Check sheet for the drawn part. Datum: minimum x, y, z corner. Units: mm. Round coordinates to 2 decimals unless told otherwise and drop trailing zeros. Write each loop counter-clockwise with the first axis right and the second up, starting at its lowest first coordinate (ties: lowest second). Pieces come first, ordered by that corner, then holes.
Item 1: Material ranges on line 1 (Z direction, x = 1.25, y = 117.15); line 2 (Y direction, x = 1.15, z = 96.36), recorded low to high.
Item 2: Cross-section at A-A on y = 117.15. Enter the section's corners in (x, z).
Item 3: Cross-section at B-B on z = 3.64. Enter the section's corners in (x, y), plus the area to 3 significant figures.
Item 4: Go/stop test with a flat-tipped pin: pin 1 Ø2 at (y, z) = (2.85, 96.36) entering from +X. Record where the tip stops, or that it passes through.
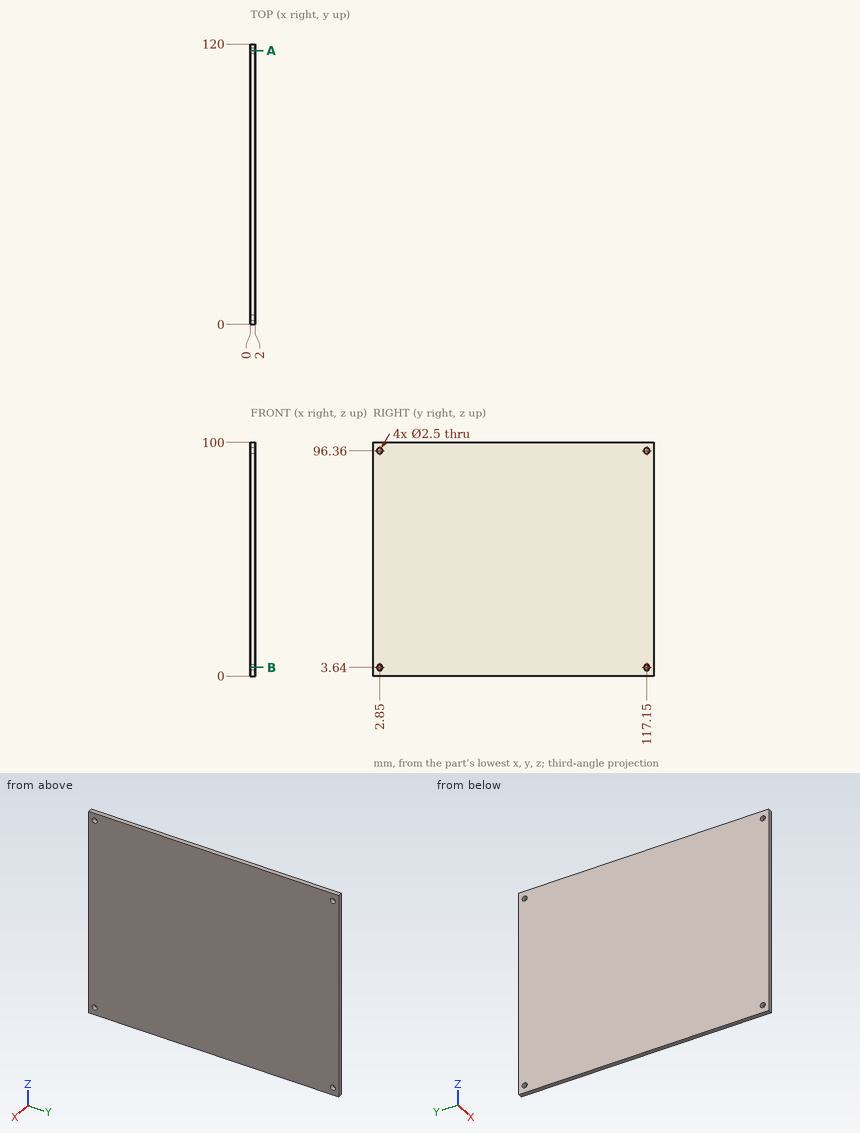
Response values:
1. line 1: z = 0 to 2.39, 4.89 to 95.11, 97.61 to 100
1. line 2: y = 0 to 1.6, 4.1 to 115.9, 118.4 to 120
2. outline: (0, 0) - (2, 0) - (2, 2.39) - (0, 2.39) - close; (0, 4.89) - (2, 4.89) - (2, 95.11) - (0, 95.11) - close; (0, 97.61) - (2, 97.61) - (2, 100) - (0, 100) - close
3. outline: (0, 0) - (2, 0) - (2, 1.6) - (0, 1.6) - close; (0, 4.1) - (2, 4.1) - (2, 115.9) - (0, 115.9) - close; (0, 118.4) - (2, 118.4) - (2, 120) - (0, 120) - close
3. area: 230 mm2
4. pin 1: passes through
